The model under review builds one solid part; all positions refer to its coordinate system, in mm. Face numbers are marked on the shaded views. A direction names the side the tool comes from. Round coordinates to 2 decimals unless told otherwise and drop trailing zeros. Write each loop counter-clockwise with the first axis right and the second up, starting at its lowest first coordinate (ties: lowest second). Pieces come first, ordered by that corner, then holes. Notation, with made-up numbers: (19.25, -8.5) - (71.25, -8.5) arc R20 ccw to (71.25, 5.5) - close; hole circle Ø3 at (-13, 19.25). An arc over 180 degrees is marked (long way). Use one line per item in the form item = value.
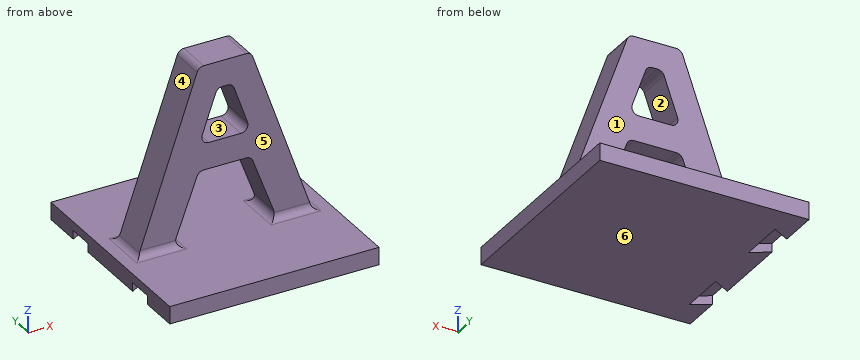
from build123d import *

# Parameters (mm, degrees)
F0_W     = 76.2
F0_H     = 76.2
F2_DEPTH = 6.35
F3_DEPTH = 6.35
F4_R     = 2.54
F6_DEPTH = 3.175


with BuildPart() as f2:
    # F0 (on Top) → F2 (new body)
    with BuildSketch(Plane.XY):
        Rectangle(F0_W, F0_H)
    extrude(amount=-F2_DEPTH)

    # F1 (on Front) → F3 (join, symmetric)
    with BuildSketch(Plane.XZ):
        Polygon((19.05, 0), (31.75, 0), (9.525, 63.5), (-9.525, 63.5), (-31.75, 0), (-19.05, 0), (-9.525, 25.4), (9.525, 25.4), align=None)
        Polygon((2.767193, 53.975), (9.434693, 34.925), (-9.434693, 34.925), (-2.767193, 53.975), align=None, mode=Mode.SUBTRACT)
    extrude(amount=F3_DEPTH, both=True)

    # F4
    f4_edges = [f2.edges().sort_by_distance(p)[0] for p in [
        (25.4, 6.35, 0),
        (19.05, 0, 0),
        (31.75, 0, 0),
        (25.4, -6.35, 0),
        (-25.4, -6.35, 0),
        (-19.05, 0, 0),
        (-25.4, 6.35, 0),
        (-31.75, 0, 0),
        (9.434693, 0, 34.925),
        (-9.434693, 0, 34.925),
        (2.767193, 0, 53.975),
        (-2.767193, 0, 53.975),
        (9.525, 0, 63.5),
        (-9.525, 0, 63.5),
        (9.525, 0, 25.4),
        (-9.525, 0, 25.4),
    ]]
    fillet(f4_edges, radius=F4_R)

    # F5 (on face) → F6 (cut)
    with BuildSketch(Plane(origin=(0, 0, -6.35), x_dir=(1, 0, 0), z_dir=(0, 0, -1))):
        Polygon((-38.1, -14.2875), (-38.1, -23.8125), (-31.75, -27.478674), (-31.75, -10.621326), align=None)
        Polygon((-31.75, 27.478674), (-38.1, 23.8125), (-38.1, 14.2875), (-31.75, 10.621326), align=None)
    extrude(amount=-F6_DEPTH, mode=Mode.SUBTRACT)


solid = f2.part
(1) Insertion check: P1, Ø1, axis at x = 1, z = 31.5, coming from the -Y side; P2, Ø1, axis at y = -16.5, z = -4, coming from the -X side. Each pin has a flat end and moves straight along its axis. Give the tip position at first contact, or say it passes through.
Geometry results:
P1 = -6.35
P2 = -31.75
(2) Add section C-C on z = 40. Write out the cut boundary in (x, y).
Geometry results:
outline = (-17.75, -6.35) - (-7.66, -6.35) - (-7.66, 6.35) - (-17.75, 6.35) - close; (7.66, -6.35) - (17.75, -6.35) - (17.75, 6.35) - (7.66, 6.35) - close
(3) Add section A-A on y = 1. Write out the cut boundary in (x, z) (3 decimals), then the cut area to 3 significant figures.
Geometry results:
outline = (-38.1, -6.35) - (38.1, -6.35) - (38.1, 0) - (33.552, 0) arc R2.54 cw to (31.155, 1.701) - (10.12, 61.799) arc R2.54 ccw to (7.723, 63.5) - (-7.723, 63.5) arc R2.54 ccw to (-10.12, 61.799) - (-31.155, 1.701) arc R2.54 cw to (-33.552, 0) - (-38.1, 0) - close; hole (-17.763, 3.432) arc R2.54 ccw to (-15.385, 0) - (15.385, 0) arc R2.54 ccw to (17.763, 3.432) - (10.143, 23.752) arc R2.54 ccw to (7.765, 25.4) - (-7.765, 25.4) arc R2.54 ccw to (-10.143, 23.752) - close; hole (-8.252, 38.304) arc R2.54 ccw to (-5.855, 34.925) - (5.855, 34.925) arc R2.54 ccw to (8.252, 38.304) - (3.363, 52.274) arc R2.54 ccw to (0.965, 53.975) - (-0.965, 53.975) arc R2.54 ccw to (-3.363, 52.274) - close
area = 2,160 mm2
(4) The part is to be moulded in two halves that separate along X. For the marked faces 1, 2, 3 and 4, say which applies: +X half, -X half, draft (parallel to the pull), parting line (faces both ways), or undercut.
Geometry results:
face_1 = draft
face_2 = undercut
face_3 = undercut
face_4 = -X half
(5) To check wall thickness, follow L1, parallel to Z at x = -18.5, y = 27.5; L2, parallel to Y at x = 17.5, z = 23. State the ranges of each line that lie inside material, in increasing order.
Geometry results:
L1 = -6.35 to 0
L2 = -6.35 to 6.35
(6) Add section D-D on y = -20. Write out the cut boundary in (x, z) (3 decimals).
Geometry results:
outline = (-38.1, -3.175) - (-31.75, -3.175) - (-31.75, -6.35) - (38.1, -6.35) - (38.1, 0) - (-38.1, 0) - close
(7) Machinability: for the marked faces 5 and 6, which of the approach directions +Z, -Z, +X, -X, +Y, -Y give a long, thin tool a straight path to every point of the face, cutting with its end or side? Answer none if there is none.
Geometry results:
face_5 = +Z, +X, -X, -Y
face_6 = -Z, +X, -X, +Y, -Y
(8) Add section B-B on x = -26.5. Write out the cut boundary in (y, z).
Geometry results:
outline = (-38.1, -6.35) - (38.1, -6.35) - (38.1, 0) - (8.89, 0) arc R2.54 cw to (6.35, 2.54) - (6.35, 15) - (-6.35, 15) - (-6.35, 2.54) arc R2.54 cw to (-8.89, 0) - (-38.1, 0) - close
